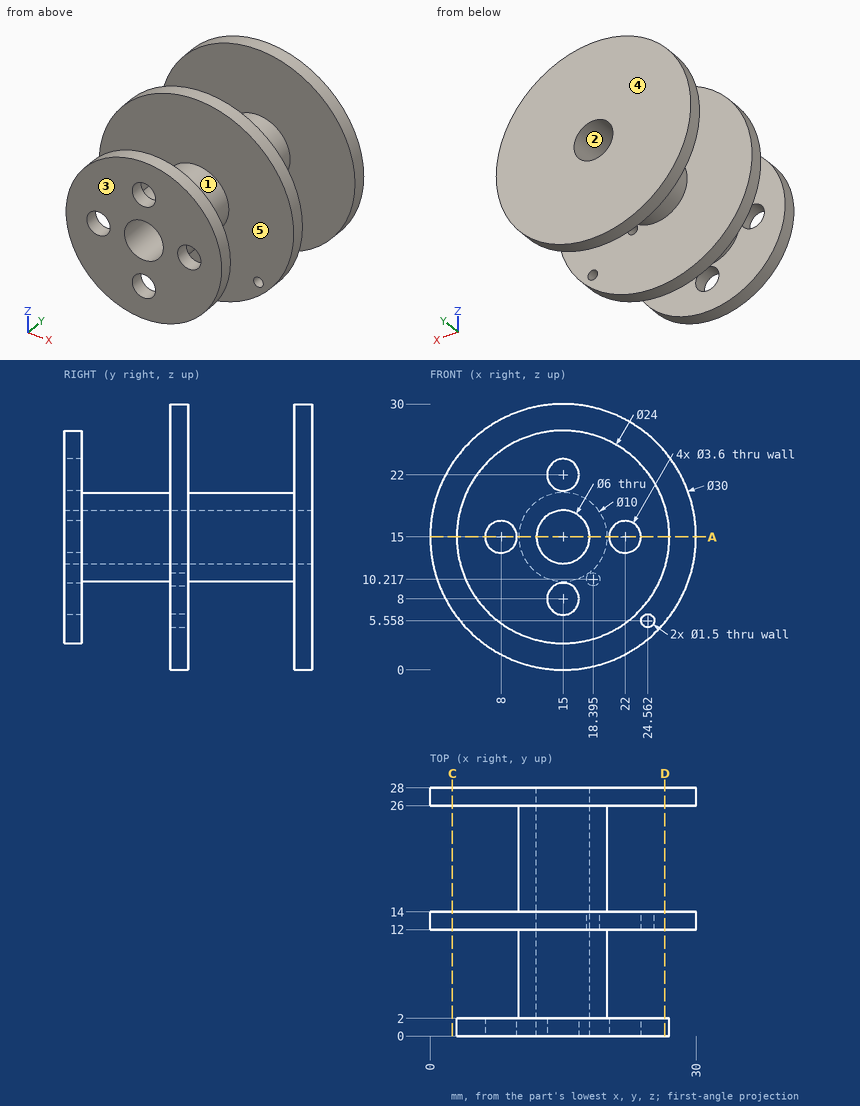
For this review, use the dimensioned drawing (mm, ordinates from the lowest corner) and the shaded views. A direction names the side the tool comes from. Give positions to 0.01 mm unless a question says otherwise; leave off trailing zeros. Loops run counter-clockwise (first coordinate to the right, second up) from the corner with the lowest first, then second, coordinate; pieces in that order, holes last. Notation, with made-up numbers: (36, -20) - (68, -20) arc R23 cw to (68, 10) - close; hole circle Ø7 at (22, 39.5). An arc over 180 degrees is marked (long way). Write each question's results on one line, items separated by ' | '.
(1) Draft analysis for pull direction Z (two halves, no side actions). For the marked faces 1, 2 and 3, state which applies: +Z half, -Z half, draft (parallel to the pull), parting line (faces both ways), or undercut.
Conclusion:
face 1: parting line | face 2: undercut | face 3: draft
(2) Take a section at D-D (x = 26.5). Give the boundary of the cut face in (y, z).
Conclusion:
outline: (0, 11.57) - (2, 11.57) - (2, 18.43) - (0, 18.43) - close; (12, 5.37) - (14, 5.37) - (14, 24.63) - (12, 24.63) - close; (26, 5.37) - (28, 5.37) - (28, 24.63) - (26, 24.63) - close
(3) For the marked faces 4 and 5, list the 3-axis set-ups (+Z, -Z, +X, -X, +Y, -Y) from which the entire face can be reached by the end or side of a thin tool; tool diameter is ignored.
Conclusion:
face 4: +Z, -Z, +X, -X, +Y | face 5: none
(4) For line 1 along Y through (x, z) = (20, 5.75); line 2 along Z through (x, y) = (15, 1.35); line 3 along Y through (x, z) = (15, 6.75), list the stretches that pass through material, from the lowest coordinate up.
Conclusion:
line 1: 0 to 2, 12 to 14, 26 to 28 | line 2: 3 to 6.2, 9.8 to 12, 18 to 20.2, 23.8 to 27 | line 3: 12 to 14, 26 to 28
(5) Take a section at A-A (z = 15). State how many separate pieces and enclosed holes the cut face has.
Conclusion:
separate pieces: 4 | enclosed holes: 0
(6) Take a section at C-C (x = 2.5). Give the boundary of the cut face in (y, z).
Conclusion:
outline: (12, 6.71) - (14, 6.71) - (14, 23.29) - (12, 23.29) - close; (26, 6.71) - (28, 6.71) - (28, 23.29) - (26, 23.29) - close
(7) For pin 1 Ø3.5 at (x, z) = (15, 15) entering from +Y; pin 2 Ø3 at (y, z) = (4, 10.5) entering from +X; pin 3 Ø12 at (x, y) = (7, 6.5) entering from +Z (1 decimal); pin 4 Ø2 at (x, y) = (17, 5.5) entering from +Z, all flat-tipped, find the tip position at first contact; note any pin that passes through.
Conclusion:
pin 1: through | pin 2: x = 19 | pin 3: z = 28.9 | pin 4: z = 19.9
